from build123d import *

# Parameters (mm, degrees)
SKETCH1_R           = 7.5
SKETCH1_R_2         = 3
BOSS_EXTRUDE1_DEPTH = 2.5
SKETCH2_W           = 80
SKETCH2_H           = 6.039840068
SKETCH2_R           = 3
BOSS_EXTRUDE2_DEPTH = 2.5
BOSS_EXTRUDE3_DEPTH = 2.5


with BuildPart() as part:
    # Sketch1 → Boss-Extrude1 (new body)
    with BuildSketch(Plane.XY):
        Circle(SKETCH1_R)
        Circle(SKETCH1_R_2, mode=Mode.SUBTRACT)
    extrude(amount=-BOSS_EXTRUDE1_DEPTH)

    # Sketch2 → Boss-Extrude2 (add)
    with BuildSketch(Plane(origin=(0, 0, -2.5), x_dir=(-1, 0, 0), z_dir=(0, 0, -1))):
        Rectangle(SKETCH2_W, SKETCH2_H)
        Circle(SKETCH2_R, mode=Mode.SUBTRACT)
    extrude(amount=-BOSS_EXTRUDE2_DEPTH)

    # Sketch4 → Boss-Extrude3 (add)
    with BuildSketch(Plane(origin=(0, 0, -2.5), x_dir=(-1, 0, 0), z_dir=(0, 0, -1))):
        with BuildLine():
            Line((27.372304228, 22.019920034), (31.255531094, 25.143820176))
            ThreePointArc((31.255531094, 25.143820176), (37.305554777, 14.745016099), (40, 3.019920034))
            Line((40, 3.019920034), (35, 3.019920034))
            ThreePointArc((35, 3.019920034), (32.601013537, 13.087927007), (27.372304228, 22.019920034))
        make_face()
        with BuildLine():
            Line((-27.372304228, 22.019920034), (-31.255531094, 25.143820176))
            ThreePointArc((-31.255531094, 25.143820176), (-37.305554777, 14.745016099), (-40, 3.019920034))
            Line((-40, 3.019920034), (-35, 3.019920034))
            ThreePointArc((-35, 3.019920034), (-32.601013537, 13.087927007), (-27.372304228, 22.019920034))
        make_face()
    extrude(amount=-BOSS_EXTRUDE3_DEPTH)


solid = part.part
The listing builds one solid part. Answer for the finished solid, in the listing's coordinates (mm). A direction names the side the tool comes from. Coordinates: 2 decimals unless noted, no trailing zeros. Write each loop counter-clockwise with the first axis right and the second up, starting at its lowest first coordinate (ties: lowest second). Pieces come first, ordered by that corner, then holes. Notation, with made-up numbers: (-15.75, 50) - (29.25, 50) arc R23 cw to (29.25, 84) - close; hole circle Ø5 at (85, 7). An arc over 180 degrees is marked (long way). Put each result on its own line as item: value.
1. The part is cut by section B-B on z = -0.5. Give the vertices of the cut face in (x, y).
Answer sheet:
outline: (-40, -3.02) - (-6.87, -3.02) arc R7.5 ccw to (6.87, -3.02) - (40, -3.02) - (40, 3.02) arc R40.11 ccw to (31.26, 25.14) - (27.37, 22.02) arc R35.13 cw to (35, 3.02) - (6.87, 3.02) arc R7.5 ccw to (-6.87, 3.02) - (-35, 3.02) arc R35.13 cw to (-27.37, 22.02) - (-31.26, 25.14) arc R40.11 ccw to (-40, 3.02) - close; hole circle Ø6 at (0, 0)
2. Find the intervals of material crossed by line 1 along X through (y, z) = (0, -1.7); line 2 along X through (y, z) = (4, -1.1); line 3 along Y through (x, z) = (-19.5, -0.8), in increasing order. Write a range as from..to.
Answer sheet:
line 1: x = -40..-3, 3..40
line 2: x = -39.91..-34.9, -6.34..6.34, 34.9..39.91
line 3: y = -3.02..3.02
3. The part is cut by section C-C on x = 0. Give the vertices of the cut face in (y, z).
Answer sheet:
outline: (-7.5, -2.5) - (-3, -2.5) - (-3, 0) - (-7.5, 0) - close; (3, -2.5) - (7.5, -2.5) - (7.5, 0) - (3, 0) - close
4. The part is cut by section A-A on y = 0. Give the vertices of the cut face in (x, z).
Answer sheet:
outline: (-40, -2.5) - (-3, -2.5) - (-3, 0) - (-40, 0) - close; (3, -2.5) - (40, -2.5) - (40, 0) - (3, 0) - close
5. Determine the mould class of faces 1 (the face through (24, -3.02, -1)), 2 (the face through (32.655, 12.953, -1.268)), 3 (the face through (40, 0, -1)), 4 (the face through (-37.243, 14.902, -1.268)) for opening direction Y: pulls with the +Y half, pulls with the -Y half, needs draft (parallel to the pull), parting line crosses it, or undercut.
Answer sheet:
face 1: pulls with the -Y half
face 2: undercut
face 3: needs draft
face 4: pulls with the +Y half
6. A tool of negligible diameter and unlimited length cuts with its end or side. For faces 5 (the face through (-23, -3.02, -1)), 6 (the face through (29.287, 23.56, -1.268)), 7 (the face through (21, 3.02, -1)), 8 (the face through (37.243, 14.902, -1.268)), 9 (the face through (0, 5, -2.5)), from which of +Z, -Z, +X, -X, +Y, -Y can it reach the whole face along a straight path? Write none if from no direction.
Answer sheet:
face 5: +Z, -Z, -X, -Y
face 6: +Z, -Z, +Y
face 7: +Z, -Z
face 8: +Z, -Z, +X, +Y
face 9: -Z, +X, -X, +Y, -Y
7. The part is cut by section D-D on x = 19.5. Give the vertices of the cut face in (y, z).
Answer sheet:
outline: (-3.02, -2.5) - (3.02, -2.5) - (3.02, 0) - (-3.02, 0) - close
8. Flat-ended cylindrical pins translate along their axes: pin 1 Ø1.2 at (x, z) = (-16.5, -1.5) entering from +Y; pin 2 Ø1.5 at (x, z) = (-4.5, -1) entering from -Y; pin 3 Ø1.5 at (x, z) = (-17.5, -1) entering from -Y; pin 4 Ø12 at (x, y) = (-17, 9.5) entering from +Z. Find the tip coordinate at first contact, or state that the pin passes through.
Answer sheet:
pin 1: stops at y = 3.02
pin 2: stops at y = -6.5
pin 3: stops at y = -3.02
pin 4: passes through
